```python
from build123d import *

# Parameters (mm, degrees)
PAD_DEPTH       = 4
POCKET_DEPTH    = 5
SKETCH005_R     = 1.8
POCKET001_DEPTH = 5
SKETCH004_W     = 4
SKETCH004_H     = 32
PAD001_DEPTH    = 11
SKETCH006_R     = 1.4
POCKET002_DEPTH = 100
POCKET003_DEPTH = 100
CHAMFER001_SIZE = 0.2


with BuildPart() as part:
    # Sketch → Pad (new body)
    with BuildSketch(Plane.XY):
        Polygon((-17, 28), (17, 28), (17, 16), (44, 16), (44, -16), (17, -16), (17, -28), (-17, -28), align=None)
    extrude(amount=PAD_DEPTH)

    # Sketch003 → Pocket (cut)
    with BuildSketch(Plane.XY.offset(4)):
        Polygon((-11, 28), (-11, -4), (0, -16), (7, -16), (7, 28), align=None)
    extrude(amount=-POCKET_DEPTH, mode=Mode.SUBTRACT)

    # Sketch005 (on Face4 of Pocket) → Pocket001 (cut)
    with BuildSketch(Plane.XY.offset(4)):
        with Locations((14, 23)):
            Circle(SKETCH005_R)
        with Locations((14, -23)):
            Circle(SKETCH005_R)
        with Locations((-14, -23)):
            Circle(SKETCH005_R)
        with Locations((-14, 23)):
            Circle(SKETCH005_R)
    extrude(amount=-POCKET001_DEPTH, mode=Mode.SUBTRACT)

    # Sketch004 (on Face2 of Pocket) → Pad001 (join)
    with BuildSketch(Plane(origin=(0, 0, 0), x_dir=(1, 0, 0), z_dir=(0, 0, -1))):
        with Locations((42, 0)):
            Rectangle(SKETCH004_W, SKETCH004_H)
        with Locations((9, 0)):
            Rectangle(SKETCH004_W, SKETCH004_H)
    extrude(amount=PAD001_DEPTH)

    # Sketch006 (on Face29 of Pad001) → Pocket002 (cut)
    with BuildSketch(Plane.YZ.offset(44)):
        with Locations((-11, -8)):
            Circle(SKETCH006_R)
        with Locations((11, -8)):
            Circle(SKETCH006_R)
    extrude(amount=-POCKET002_DEPTH, mode=Mode.SUBTRACT)

    # Sketch007 (on Face33 of Pocket002) → Pocket003 (cut)
    with BuildSketch(Plane.YZ.offset(44)):
        with BuildLine():
            Line((8, -7.650166), (8, -4.2))
            Line((8, -4.2), (-8, -4.2))
            Line((-8, -4.2), (-8, -7.650166))
            ThreePointArc((-8, -7.650166), (0, -26.2), (8, -7.650166))
        make_face()
    extrude(amount=-POCKET003_DEPTH, mode=Mode.SUBTRACT)

    # Chamfer001
    chamfer001_edges = [part.edges().sort_by_distance(p)[0] for p in [
        (-15.8, 23, 4),
        (-15.8, -23, 4),
        (12.2, -23, 4),
        (12.2, 23, 4),
    ]]
    chamfer(chamfer001_edges, length=CHAMFER001_SIZE)


solid = part.part
```
The listing builds one solid part. Answer for the finished solid, in the listing's coordinates (mm). A direction names the side the tool comes from. Round coordinates to 2 decimals unless told otherwise and drop trailing zeros. Write each loop counter-clockwise with the first axis right and the second up, starting at its lowest first coordinate (ties: lowest second). Pieces come first, ordered by that corner, then holes. Notation, with made-up numbers: (4, 54) -> (58, 54) arc R30 ccw to (58, 77) -> close; hole circle Ø1 at (11.25, 58.25). An arc over 180 degrees is marked (long way). Use CSV: the item, a comma, the result in double quotes. Start each with the question number.
(1) Section B-B on y = 4 is taken. Give the vertices of the cut face in (x, z), then the cut area to 3 significant figures.
(2) The mould has two halves that part along Z. Classify faces 5 (the face through (42, -13, -11)), 6 (the face through (9.03, 9.89, -8.85)), 7 (the face through (-11, 12, 2)): released by +Z, released by -Z, zero draft, split by the parting line, or undercut.
(3) Section D-D on x = -14 is taken. Give the vertices of the cut face in (y, z), then the cut area to 3 significant figures.
(4) Consider L1, parallel to Y at x = 14, z = 2.5; L2, parallel to X at y = -2.5, z = -3.5; L3, parallel to X at y = -2, z = 2. Determine where each line is inside the solid, lowest interval first. Write a range as from..to.
(5) Which of the six approach directions +Z, -Z, +X, -X, +Y, -Y give full straight-line access (tool end or side, diameter ignored) to faces 1 (the face through (34, 16, 1)), 2 (the face through (9, 0, -4.2)), 3 (the face through (-5.577, -9.916, 2.028)), 4 (the face through (9, 16, -5))?
(6) Section A-A on y = 11 is taken. Give the vertices of the cut face in (x, z), then the cut area to 3 significant figures.
(7) Each of these flat-tipped pins is pushed along its axis until it touches: pin 1 (5 mm diameter, centred on y = 16, z = -7, fed in from -X); pin 2 (3.5 mm diameter, centred on y = -11, z = -8, fed in from +X); pin 3 (1.2 mm diameter, centred on x = 9.5, z = -7.5, fed in from +Y); pin 4 (3 mm diameter, centred on y = 21.5, z = 2.5, fed in from +X). Where does it stop, or does it pass through?
(8) Section C-C on z = -1.5 is taken. Give the vertices of the cut face in (x, y).
A:
1,outline,"(-17, 0) -> (-11, 0) -> (-11, 4) -> (-17, 4) -> close; (7, -4.2) -> (11, -4.2) -> (11, 0) -> (40, 0) -> (40, -4.2) -> (44, -4.2) -> (44, 4) -> (7, 4) -> close"
1,area,"206 mm²"
2,face 5,"released by -Z"
2,face 6,"undercut"
2,face 7,"zero draft"
3,outline,"(-28, 0) -> (-24.8, 0) -> (-24.8, 3.8) -> (-25, 4) -> (-28, 4) -> close; (-21.2, 0) -> (21.2, 0) -> (21.2, 3.8) -> (21, 4) -> (-21, 4) -> (-21.2, 3.8) -> close; (24.8, 0) -> (28, 0) -> (28, 4) -> (25, 4) -> (24.8, 3.8) -> close"
3,area,"195 mm²"
4,L1,"y = -28..-24.8, -21.2..21.2, 24.8..28"
4,L2,"x = 7..11, 40..44"
4,L3,"x = -17..-11, 7..44"
5,face 1,"+Z, -Z, +X, +Y"
5,face 2,"-Z, +X, -X"
5,face 3,"+Z, -Z, +Y"
5,face 4,"-Z, +X, -X, +Y"
6,outline,"(-17, 0) -> (-11, 0) -> (-11, 4) -> (-17, 4) -> close; (7, -11) -> (11, -11) -> (11, -9.4) -> (7, -9.4) -> close; (7, -6.6) -> (11, -6.6) -> (11, 0) -> (40, 0) -> (40, -6.6) -> (44, -6.6) -> (44, 4) -> (7, 4) -> close; (40, -11) -> (44, -11) -> (44, -9.4) -> (40, -9.4) -> close"
6,area,"238 mm²"
7,pin 1,"stops at x = 7"
7,pin 2,"stops at x = 44"
7,pin 3,"stops at y = 16"
7,pin 4,"stops at x = 17"
8,outline,"(7, -16) -> (11, -16) -> (11, 16) -> (7, 16) -> close; (40, -16) -> (44, -16) -> (44, 16) -> (40, 16) -> close"
